The model under review builds one solid part; all positions refer to its coordinate system, in mm. A direction names the side the tool comes from. Coordinates: 2 decimals unless noted, no trailing zeros. Order: outer loops, then holes, each group sorted by start corner. A loop starts at its lowest first (then second) coordinate and runs counter-clockwise, first axis right, second up. Notation, with made-up numbers: (46.25, 15.25) - (57.25, 15.25) arc R32 ccw to (57.25, 45.25) - close; hole circle Ø3 at (81.25, 61.25). An arc over 180 degrees is marked (long way). Answer in a Markdown table with one row per item.
```python
from build123d import *

# Parameters (mm, degrees)
SKETCH1_W                 = 19.05
SKETCH1_H                 = 19.05
SKETCH1_W_2               = 15.875
SKETCH1_H_2               = 15.875
BOSS_EXTRUDE1_DEPTH       = 328.6633
SKETCH2_R                 = 1.7145
CUT_EXTRUDE1_DEPTH        = 330.352687695
LPATTERN1_COUNT           = 5
LPATTERN1_PITCH           = 25.4
LPATTERN2_COUNT           = 2
LPATTERN2_PITCH           = 177.8
LPATTERN2_COPY_1_SKETCH_R = 1.7145
LPATTERN2_COPY_1_DEPTH    = 330.352687695
LPATTERN2_COPY_2_SKETCH_R = 1.7145
LPATTERN2_COPY_2_DEPTH    = 330.352687695
LPATTERN2_COPY_3_SKETCH_R = 1.7145
LPATTERN2_COPY_3_DEPTH    = 330.352687695
LPATTERN2_COPY_4_SKETCH_R = 1.7145
LPATTERN2_COPY_4_DEPTH    = 330.352687695


with BuildPart() as part:
    # Sketch1 → Boss-Extrude1 (new, symmetric)
    with BuildSketch(Plane.ZX):
        Rectangle(SKETCH1_W, SKETCH1_H)
        Rectangle(SKETCH1_W_2, SKETCH1_H_2, mode=Mode.SUBTRACT)
    extrude(amount=BOSS_EXTRUDE1_DEPTH, both=True)

    # Sketch2 → Cut-Extrude1 (cut, through all)
    with BuildSketch(Plane.XY.offset(9.525)):
        with Locations((0, -74.6633)):
            Circle(SKETCH2_R)
    cut_extrude1 = extrude(amount=-CUT_EXTRUDE1_DEPTH, mode=Mode.SUBTRACT)

    # LPattern1: Cut-Extrude1 ×5
    with Locations(*[(0, i * LPATTERN1_PITCH, 0) for i in range(1, LPATTERN1_COUNT)]):
        add(cut_extrude1, mode=Mode.SUBTRACT)

    # LPattern2: Cut-Extrude1 ×2
    with Locations(*[(0, i * LPATTERN2_PITCH, 0) for i in range(1, LPATTERN2_COUNT)]):
        add(cut_extrude1, mode=Mode.SUBTRACT)

    # LPattern2 copy 1 sketch → LPattern2 copy 1 (cut, through all)
    with BuildSketch(Plane(origin=(0, 203.2, 9.525), x_dir=(1, 0, 0), z_dir=(0, 0, 1))):
        with Locations((0, -74.6633)):
            Circle(LPATTERN2_COPY_1_SKETCH_R)
    extrude(amount=-LPATTERN2_COPY_1_DEPTH, mode=Mode.SUBTRACT)

    # LPattern2 copy 2 sketch → LPattern2 copy 2 (cut, through all)
    with BuildSketch(Plane(origin=(0, 228.6, 9.525), x_dir=(1, 0, 0), z_dir=(0, 0, 1))):
        with Locations((0, -74.6633)):
            Circle(LPATTERN2_COPY_2_SKETCH_R)
    extrude(amount=-LPATTERN2_COPY_2_DEPTH, mode=Mode.SUBTRACT)

    # LPattern2 copy 3 sketch → LPattern2 copy 3 (cut, through all)
    with BuildSketch(Plane(origin=(0, 254, 9.525), x_dir=(1, 0, 0), z_dir=(0, 0, 1))):
        with Locations((0, -74.6633)):
            Circle(LPATTERN2_COPY_3_SKETCH_R)
    extrude(amount=-LPATTERN2_COPY_3_DEPTH, mode=Mode.SUBTRACT)

    # LPattern2 copy 4 sketch → LPattern2 copy 4 (cut, through all)
    with BuildSketch(Plane(origin=(0, 279.4, 9.525), x_dir=(1, 0, 0), z_dir=(0, 0, 1))):
        with Locations((0, -74.6633)):
            Circle(LPATTERN2_COPY_4_SKETCH_R)
    extrude(amount=-LPATTERN2_COPY_4_DEPTH, mode=Mode.SUBTRACT)


solid = part.part
```
Item 1: We need section B-B, the plane y = 54.5. Write out the cut boundary in (x, z) (1 decimal).
Check values:
| item | result |
|---|---|
| outline | (-9.5, -9.5) - (9.5, -9.5) - (9.5, 9.5) - (-9.5, 9.5) - close; hole (-7.9, -7.9) - (7.9, -7.9) - (7.9, 7.9) - (-7.9, 7.9) - close |
Item 2: Tool access review of faces 1 (the face through (7.938, 5, 0)), 2 (the face through (0, 328.663, -9)): name each direction out of +Z, -Z, +X, -X, +Y, -Y from which nothing blocks a thin tool from reaching the whole face with its end or side.
Check values:
| item | result |
|---|---|
| face 1 | +Y, -Y |
| face 2 | +Z, -Z, +X, -X, +Y |
Item 3: To check wall thickness, follow line 1 (X direction, y = -74, z = -2) (1 decimal). State the ranges of the line that lie inside material, in increasing order. Write a range as from..to.
Check values:
| item | result |
|---|---|
| line 1 | -9.5..-7.9, 7.9..9.5 |
Item 4: We need section A-A, the plane z = 1.75. Write out the cut boundary in (x, y) (1 decimal).
Check values:
| item | result |
|---|---|
| outline | (-9.5, -328.7) - (-7.9, -328.7) - (-7.9, 328.7) - (-9.5, 328.7) - close; (7.9, -328.7) - (9.5, -328.7) - (9.5, 328.7) - (7.9, 328.7) - close |
Item 5: Mouldability with a two-part tool opening along Z and no side actions: class faces 3 (the face through (-9.525, 5, 0)), 4 (the face through (0, 5, 7.938)), 5 (the face through (0, 5, -9.525)), 6 (the face through (0, 5, 9.525)) as +Z half, -Z half, draft (parallel to the pull), parting line (faces both ways), or undercut.
Check values:
| item | result |
|---|---|
| face 3 | draft |
| face 4 | undercut |
| face 5 | -Z half |
| face 6 | +Z half |
Item 6: Clearance check with flat-ended pins moving along their axes: pin 1 Ø3 at (x, y) = (0, -23.86) entering from +Z; pin 2 Ø5.5 at (x, y) = (0, -49.26) entering from +Z (3 decimals). State where each tip first meets the part, or that it passes through.
Check values:
| item | result |
|---|---|
| pin 1 | through |
| pin 2 | z = 9.525 |
